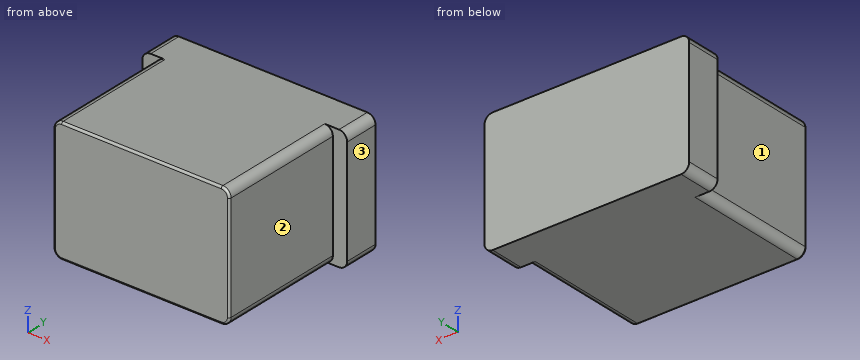
Autodesk Inventor part; units mm, degrees
ref_plane "YZ Plane" through (0, 0, 0) normal (1, 0, 0) x (0, 1, 0)
ref_plane "XZ Plane" through (0, 0, 0) normal (0, 1, 0) x (-1, 0, 0)
ref_plane "XY Plane" through (0, 0, 0) normal (0, 0, 1) x (1, 0, 0)
sketch "Sketch1" plane through (0, 0, 0) normal (0, 0, 1) x (1, 0, 0)
  line L0 (-136.525, 0) -> (136.525, 0)
  line L1 (136.525, 0) -> (136.525, 196.85)
  line L2 (136.525, 196.85) -> (-136.525, 196.85)
  line L3 (-136.525, 196.85) -> (-136.525, 0)
  line L4 (-158.75, 196.85) -> (158.75, 196.85)
  line L5 (158.75, 196.85) -> (158.75, 250.825)
  line L6 (158.75, 250.825) -> (-158.75, 250.825)
  line L7 (-158.75, 250.825) -> (-158.75, 196.85)
  point P0 (0, 0)
  point P1 (0, 196.85)
  point P2 (0, 0)
  dimension "d0" = 250.825
  dimension "d1" = 317.5
  dimension "d2" = 196.85
  dimension "d3" = 273.05
extrude "Extrusion1" add sketch "Sketch1" along normal blind 190.5
fillet "Fillet1" radius 3.175 4 edges at (0, 0, 190.5) (136.525, 0, 95.25) (0, 0, 0) (-136.525, 0, 95.25)
fillet "Fillet1" radius 12.7 8 edges at (136.525, 98.425, 190.5) (136.525, 98.425, 0) (-136.525, 98.425, 190.5) (-136.525, 98.425, 0) (-158.75, 223.8375, 190.5) (-158.75, 223.8375, 0) (158.75, 223.8375, 190.5) (158.75, 223.8375, 0)
properties part number "battery"
Build history of the part. All positions in model axes, mm. Face numbers are marked on the shaded views. A direction names the side the tool comes from. Round coordinates to 2 decimals unless told otherwise and drop trailing zeros. Order: outer loops, then holes, each group sorted by start corner. A loop starts at its lowest first (then second) coordinate and runs counter-clockwise, first axis right, second up. Notation, with made-up numbers: M -40,-5 L -5,-5 A23 ccw -5,11 Z; hole C 85,-8.75 d1. An arc over 180 degrees is marked long. Use CSV: the item, a comma, the result in double quotes. Start each with the question number.
(1) Flat gauge pins, fed straight in: P1, Ø1.5, axis at x = 117.5, y = 87, coming from the -Z side; P2, Ø8, axis at y = 60, z = 84.5, coming from the +X side (3 decimals); P3, Ø1.5, axis at y = 109.5, z = 38, coming from the -X side (3 decimals). Where does each tip first touch, or does it go through?
(2) Tool access for the marked faces 1, 2 and 3: list every direction of +Z, -Z, +X, -X, +Y, -Y with a clear straight run to the whole face (end or side of a thin tool).
(3) Cut at B-B on z = 17. List the corners of the cut face in (x, y) (3 decimals), then the cut area to 3 significant figures.
(4) Cut at A-A on y = 128. List the corners of the cut face in (x, z) (3 decimals), then the cut area to 3 significant figures.
(5) Drill centre lines: probe 1 along X at (y, z) = (89.5, 141) (3 decimals); probe 2 along Y at (x, z) = (135, 53) (3 decimals). Where is each one in solid material? Low to high.
Findings:
1,P1,"stops at z = 0"
1,P2,"stops at x = 136.525"
1,P3,"stops at x = -136.525"
2,face 1,"+Z, -Z, -X, -Y"
2,face 2,"+Z, -Z, +X, -Y"
2,face 3,"+Z, -Z, +X, +Y, -Y"
3,outline,"M -158.75,196.85 L -136.525,196.85 L -136.525,3.175 A3.175 ccw -133.35,0 L 133.35,0 A3.175 ccw 136.525,3.175 L 136.525,196.85 L 158.75,196.85 L 158.75,250.825 L -158.75,250.825 Z"
3,area,"70,900 mm^2"
4,outline,"M -136.525,12.7 A12.7 ccw -123.825,0 L 123.825,0 A12.7 ccw 136.525,12.7 L 136.525,177.8 A12.7 ccw 123.825,190.5 L -123.825,190.5 A12.7 ccw -136.525,177.8 Z"
4,area,"51,900 mm^2"
5,probe 1,"x = -136.525 to 136.525"
5,probe 2,"y = 0.462 to 250.825"
